Answer from the drawing. Dimensions are ordinates in mm from the lowest x, y and z of the part. Give positions to 0.01 mm unless a question says otherwise; leave off trailing zeros. Write each loop counter-clockwise with the first axis right and the second up, starting at its lowest first coordinate (ties: lowest second). Pieces come first, ordered by that corner, then holes. Notation, with made-up numbers: M -17.75,69 L 18.25,69 A34 ccw 18.25,101 Z; hole C 33,-28 d5. An arc over 180 degrees is marked long. Put each result on its own line as item: value.
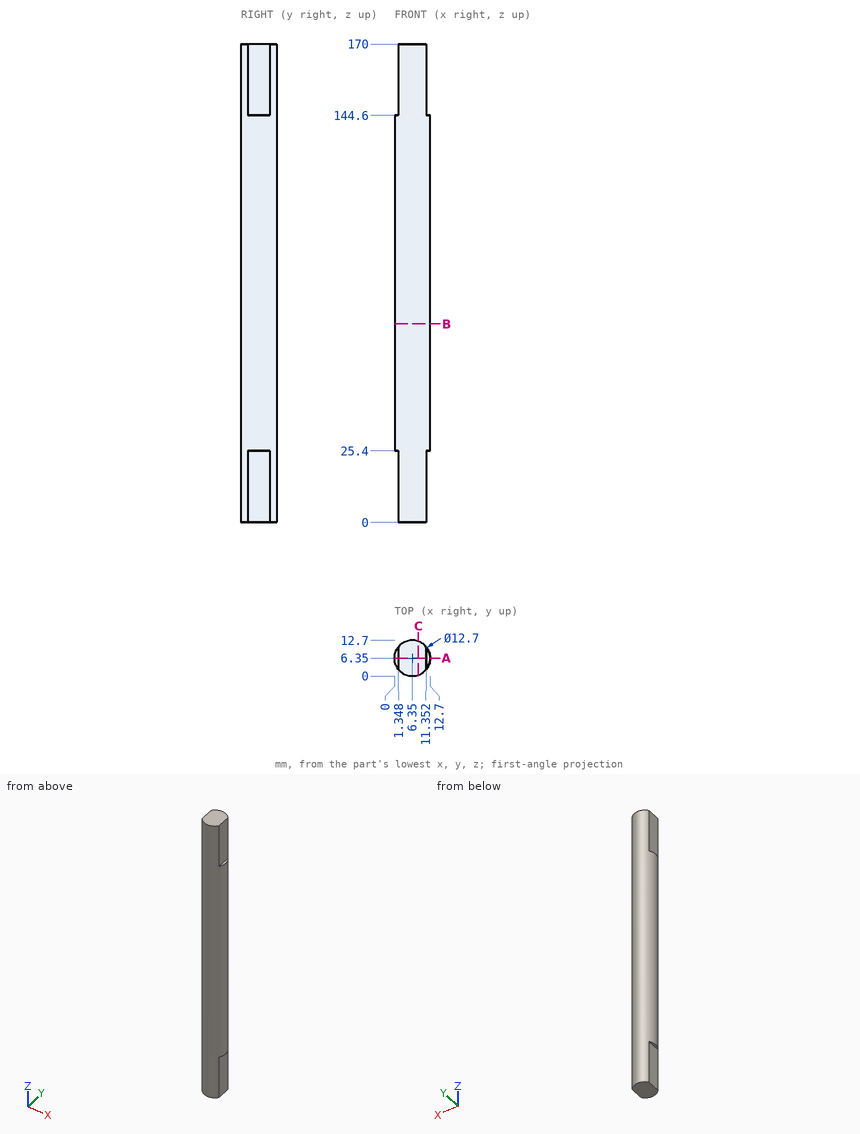
(1) Section C-C on x = 8.5 is taken. Determine the outline of the cut face in (y, z) (3 decimals), and give its area (3 significant figures).
Result:
outline: M 0.375,0 L 12.325,0 L 12.325,170 L 0.375,170 Z
area: 2,030 mm²
(2) Straight lines are drawn through the part: line 1 along X through (y, z) = (6.25, 141.5); line 2 along Y through (x, z) = (5.75, 133.5); line 3 along X through (y, z) = (7.5, 24). For each, find the intervals that lie inside material, in ascending order. Write a range as from..to.
Result:
line 1: x = 0..12.7
line 2: y = 0.03..12.67
line 3: x = 1.35..11.35
(3) Section A-A on y = 6.35 is taken. Determine the outline of the cut face in (x, z).
Result:
outline: M 0,25.4 L 1.35,25.4 L 1.35,0 L 11.35,0 L 11.35,25.4 L 12.7,25.4 L 12.7,144.6 L 11.35,144.6 L 11.35,170 L 1.35,170 L 1.35,144.6 L 0,144.6 Z
(4) Given pin 1 Ø4 at (y, z) = (6.5, 8.5) entering from +X; pin 2 Ø6 at (y, z) = (9.5, 120) entering from +X; pin 3 Ø2.5 at (y, z) = (7.5, 153.5) entering from -X, each flat-ended and moving along its own axis, determine where each tip first touches the part or whether it passes through.
Result:
pin 1: stops at x = 11.35
pin 2: stops at x = 12.7
pin 3: stops at x = 1.35
(5) Section B-B on z = 70.5 is taken. Determine the outline of the cut face in (x, y), and give its area (3 significant figures).
Result:
outline: C 6.35,6.35 d12.7
area: 127 mm²
